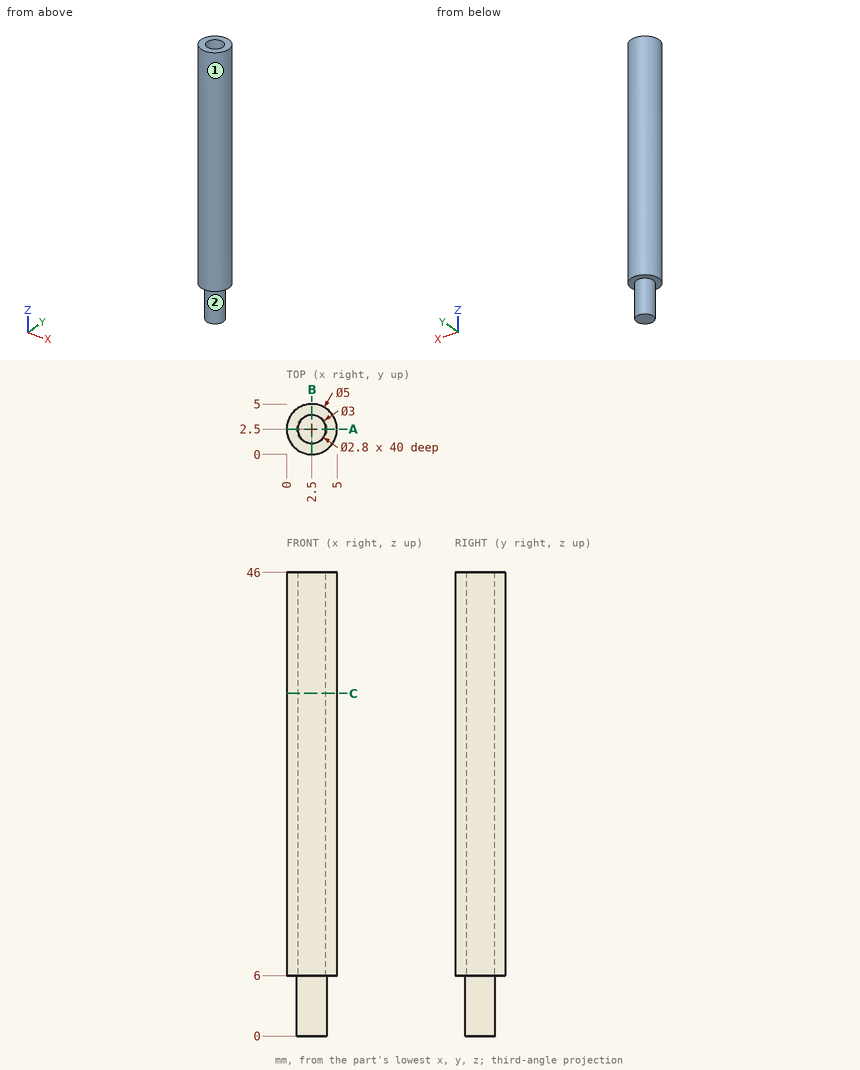
Drawing for the job (mm, zero at the part's lowest x, y, z). A direction names the side the tool comes from. Coordinates: 2 decimals unless noted, no trailing zeros. Write each loop counter-clockwise with the first axis right and the second up, starting at its lowest first coordinate (ties: lowest second). Pieces come first, ordered by that corner, then holes. Notation, with made-up numbers: (9, -21) - (45, -21) arc R24 ccw to (45, 15) - close; hole circle Ø9 at (10, 9). An arc over 180 degrees is marked (long way). Write each question's results on one line, items separated by ' | '. Start each with the question number.
1) 3-axis set-ups, long thin cutter, end or side, ignore diameter. For the marked faces 1 and 2: which of +Z, -Z, +X, -X, +Y, -Y reach the whole face in a straight line?
2) Cut at A-A (y = 2.5). Write the cut outline in (x, z).
3) Probe line 1 along Y through (x, z) = (2.5, 24); line 2 along Z through (x, y) = (2, 2.8); line 3 along X through (y, z) = (4.5, 13.5). List the from-to ranges inside material, lowest first. Write a range as from..to.
4) Flat gauge pin, fed straight in: P1, Ø1.5, axis at y = 4.5, z = 28, coming from the -X side. Where does the tip first touch, or does it go through?
5) Cut at C-C (z = 34). Write the cut outline in (x, y).
Returned:
1) face 1: +Z, -Z | face 2: -Z
2) outline: (0, 6) - (1, 6) - (1, 0) - (4, 0) - (4, 6) - (5, 6) - (5, 46) - (3.9, 46) - (3.9, 6) - (1.1, 6) - (1.1, 46) - (0, 46) - close
3) line 1: 0..1.1, 3.9..5 | line 2: 0..6 | line 3: 1..4
4) P1: x = 0.33
5) outline: circle Ø5 at (2.5, 2.5); hole circle Ø2.8 at (2.5, 2.5)
